from build123d import *

# Parameters (mm, degrees)
BOSS_EXTRU_1_DEPTH      = 10
ESQUISSE2_R             = 1.5
ENL_V_MAT_EXTRU_1_DEPTH = 35.183235498


with BuildPart() as part:
    # Esquisse1 → Boss.-Extru.1 (new body)
    with BuildSketch(Plane.XY):
        with BuildLine():
            Line((0.481491326, 8.144757028), (-7.518508674, 8.144757028))
            ThreePointArc((-7.518508674, 8.144757028), (-8.932722237, 8.730543466), (-9.518508674, 10.144757028))
            Line((-9.518508674, 10.144757028), (-9.518508674, 19.144757028))
            Line((-9.518508674, 19.144757028), (-13.518508674, 19.144757028))
            Line((-13.518508674, 19.144757028), (-13.518508674, -25.855242972))
            Line((-13.518508674, -25.855242972), (-8.518508674, -25.855242972))
            Line((-8.518508674, -25.855242972), (-8.518508674, -10.855242972))
            ThreePointArc((-8.518508674, -10.855242972), (-7.932722237, -9.441029409), (-6.518508674, -8.855242972))
            Line((-6.518508674, -8.855242972), (-0.518508674, -8.855242972))
            ThreePointArc((-0.518508674, -8.855242972), (0.895704888, -9.441029409), (1.481491326, -10.855242972))
            Line((1.481491326, -10.855242972), (1.481491326, -25.855242972))
            Line((1.481491326, -25.855242972), (6.481491326, -25.855242972))
            Line((6.481491326, -25.855242972), (6.481491326, 19.144757028))
            Line((6.481491326, 19.144757028), (2.481491326, 19.144757028))
            Line((2.481491326, 19.144757028), (2.481491326, 10.144757028))
            ThreePointArc((2.481491326, 10.144757028), (1.895704888, 8.730543466), (0.481491326, 8.144757028))
        make_face()
    extrude(amount=BOSS_EXTRU_1_DEPTH)

    # Esquisse2 → Enlèv. mat.-Extru.1 (cut, through all)
    with BuildSketch(Plane.ZY.offset(13.518508674)):
        with BuildLine():
            ThreePointArc((10, -20.855242972), (8.535533906, -24.390776877), (5, -25.855242972))
            Line((5, -25.855242972), (10, -25.855242972))
            Line((10, -25.855242972), (10, -20.855242972))
        make_face()
        with BuildLine():
            ThreePointArc((5, -25.855242972), (1.464466094, -24.390776877), (0, -20.855242972))
            Line((0, -20.855242972), (0, -25.855242972))
            Line((0, -25.855242972), (5, -25.855242972))
        make_face()
        with Locations((5, -20.855242972)):
            Circle(ESQUISSE2_R)
        with BuildLine():
            Line((10, 19.144757028), (5, 19.144757028))
            ThreePointArc((5, 19.144757028), (8.535533906, 17.680290934), (10, 14.144757028))
            Line((10, 14.144757028), (10, 19.144757028))
        make_face()
        with BuildLine():
            Line((0, 19.144757028), (0, 14.144757028))
            ThreePointArc((0, 14.144757028), (1.464466094, 17.680290934), (5, 19.144757028))
            Line((5, 19.144757028), (0, 19.144757028))
        make_face()
        with Locations((5, 14.144757028)):
            Circle(ESQUISSE2_R)
        with Locations((5, -14.195242972)):
            Circle(ESQUISSE2_R)
    extrude(amount=-ENL_V_MAT_EXTRU_1_DEPTH, mode=Mode.SUBTRACT)


solid = part.part
Build history of the part. All positions in model axes, mm. A direction names the side the tool comes from. Coordinates: 2 decimals unless noted, no trailing zeros. Order: outer loops, then holes, each group sorted by start corner. A loop starts at its lowest first (then second) coordinate and runs counter-clockwise, first axis right, second up. Notation, with made-up numbers: (76, 84) - (93, 84) arc R19 cw to (93, 101) - close; hole circle Ø7 at (5.25, 21). An arc over 180 degrees is marked (long way). Write each question's results on one line, items separated by ' | '. Start each with the question number.
Item 1: Band-saw the part on C-C on z = 1.5. Write the cut outline in (x, y), and give its area (3 significant figures).
Item 2: Mould opens along Y. For faces 4 (the face through (-4, -3, 0)), 5 (the face through (-11.55, 12.68, 4.67)), 6 (the face through (-8.9, 8.7, 4.9)), 7 (the face through (-11.054, -12.93, 5.806)) say: released by +Y, released by -Y, zero draft, split by the parting line, or undercut.
Item 3: Band-saw the part on D-D on z = 5.5. State how many separate pieces and enclosed holes the cut face has, and give its area (3 significant figures).
Item 4: Band-saw the part on A-A on y = -17. Write the cut outline in (x, z).
Item 5: Flat gauge pins, fed straight in: pin 1 (5 mm diameter, centred on x = -4, z = 3.5, fed in from +Y); pin 2 (1.8 mm diameter, centred on y = 14.14, z = 5, fed in from -X); pin 3 (5 mm diameter, centred on x = -4, z = 6.5, fed in from -Y); pin 4 (6 mm diameter, centred on x = -1, z = 8.5, fed in from -Y). Where does each tip first touch, or does it go through?
Item 6: Band-saw the part on B-B on x = 4. Write the cut outline in (y, z).
Item 7: Tool access for faces 1 (the face through (-3, 8.145, 5)), 2 (the face through (-4, -8.855, 5)), 3 (the face through (-13.519, -3, 5)): list every direction of +Z, -Z, +X, -X, +Y, -Y with a clear straight run to the whole face (end or side of a thin tool).
Item 8: Wall check: probe 1 along Y at (x, z) = (-10.25, 5); probe 2 along X at (y, z) = (-11.5, 4.5); probe 3 along Y at (x, z) = (4.75, 6.25). Give the ranges that are in metal, low to high. Write a range as [from, to].
Numbers:
1) outline: (-13.52, -24.43) - (-8.52, -24.43) - (-8.52, -10.86) arc R2 cw to (-6.52, -8.86) - (-0.52, -8.86) arc R2 cw to (1.48, -10.86) - (1.48, -24.43) - (6.48, -24.43) - (6.48, 17.72) - (2.48, 17.72) - (2.48, 10.14) arc R2 cw to (0.48, 8.14) - (-7.52, 8.14) arc R2 cw to (-9.52, 10.14) - (-9.52, 17.72) - (-13.52, 17.72) - close | area: 576 mm^2
2) face 4: zero draft | face 5: undercut | face 6: released by +Y | face 7: undercut
3) separate pieces: 7 | enclosed holes: 0 | area: 522 mm^2
4) outline: (-13.52, 0) - (-8.52, 0) - (-8.52, 10) - (-13.52, 10) - close; (1.48, 0) - (6.48, 0) - (6.48, 10) - (1.48, 10) - close
5) pin 1: y = 8.14 | pin 2: through | pin 3: y = -8.86 | pin 4: y = -25.51
6) outline: (-20.86, 0) - (14.14, 0) arc R5 ccw to (14.14, 10) - (-20.86, 10) arc R5 ccw to start; hole circle Ø3 at (-20.86, 5); hole circle Ø3 at (-14.2, 5); hole circle Ø3 at (14.14, 5)
7) face 1: +Z, -Z, +Y | face 2: +Z, -Z, -Y | face 3: +Z, -Z, -X, +Y, -Y
8) probe 1: [-25.86, -22.36], [-19.36, -15.7], [-12.7, 12.64], [15.64, 19.14] | probe 2: [-13.52, -8.52], [1.48, 6.48] | probe 3: [-25.7, -21.68], [-20.03, -15.02], [-13.37, 13.32], [14.97, 18.99]
